```python
from build123d import *

# Parameters (mm, degrees)
F0_R     = 63.75
F1_DEPTH = 20
F2_R     = 55
F3_DEPTH = 25


with BuildPart() as f1:
    # F0 (on Top) → F1 (new body)
    with BuildSketch(Plane.XY):
        Circle(F0_R)
    extrude(amount=F1_DEPTH)


with BuildPart() as f3:
    # F2 (on Top) → F3 (new body)
    with BuildSketch(Plane.XY):
        with Locations((-173.995957, -105.135567)):
            Circle(F2_R)
    extrude(amount=F3_DEPTH)


with BuildPart() as f3_1:
    # F4: moved
    add(f3.part.moved(Location((173.8, 105.1, -2.2))))


with BuildPart() as f1_1:
    add(f1.part)

    # F5: cut F3
    add(f3_1.part, mode=Mode.SUBTRACT)


solid = f1_1.part
```
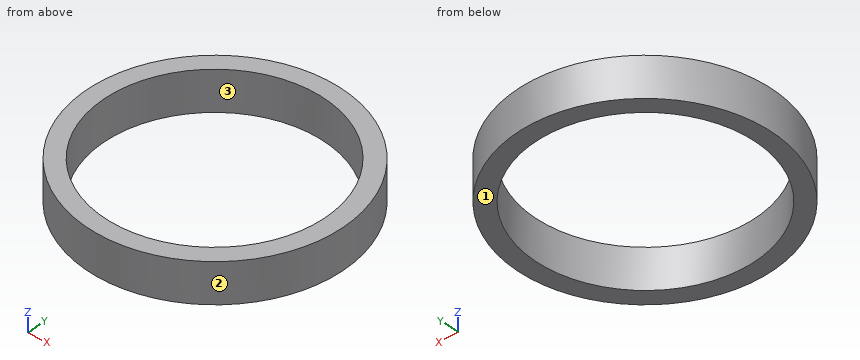
Check sheet for the modelled part. Datum: model origin and axes. Units: mm. Face numbers are marked on the shaded views. Coordinates: 2 decimals unless noted, no trailing zeros. Order: outer loops, then holes, each group sorted by start corner. A loop starts at its lowest first (then second) coordinate and runs counter-clockwise, first axis right, second up. Notation, with made-up numbers: (64.25, -5.5) -> (110.25, -5.5) arc R18 ccw to (110.25, 20.5) -> close; hole circle Ø9 at (34.25, 62.25). An arc over 180 degrees is marked (long way). Write item = value, one per line. Start each with the question number.
1) Cross-section at B-B (y = 29). Enter the section's corners in (x, z).
2) Go/stop test with flat-tipped pins: P1, Ø5, axis at y = -16.5, z = 17, coming from the +X side; P2, Ø2, axis at x = 43.5, z = 12, coming from the +Y side; P3, Ø5, axis at x = -13, z = 9.5, coming from the -Y side. Record where each tip stops, or that it passes through.
3) Cross-section at C-C (z = 9.25). Enter the section's corners in (x, y), then the cut area to 3 significant figures.
4) Mould release check, pull along Y, two halves, no side actions. Record for the marked faces 1, 2 and 3: +Y half, -Y half, draft (parallel to the pull), parting line (faces both ways), or undercut.
5) Cross-section at A-A (x = -26). Enter the section's corners in (y, z).
6) Material ranges on L1, parallel to Y at x = -1, z = 6.5; L2, parallel to X at y = 1.5, z = 2.25; L3, parallel to X at y = -43, z = 3.75, recorded low to high.
Ans:
q1.outline = (-56.77, 0) -> (-46.91, 0) -> (-46.91, 20) -> (-56.77, 20) -> close; (46.52, 0) -> (56.77, 0) -> (56.77, 20) -> (46.52, 20) -> close
q2.P1 = 62.19
q2.P2 = 47.52
q2.P3 = -62.88
q3.outline = circle Ø127.5 at (0, 0); hole circle Ø110 at (-0.2, -0.04)
q3.area = 3,260 mm²
q4.face_1 = draft
q4.face_2 = parting line
q4.face_3 = undercut
q5.outline = (-58.21, 0) -> (-48.61, 0) -> (-48.61, 20) -> (-58.21, 20) -> close; (48.54, 0) -> (58.21, 0) -> (58.21, 20) -> (48.54, 20) -> close
q6.L1 = -63.74 to -55.03, 54.96 to 63.74
q6.L2 = -63.73 to -55.17, 54.78 to 63.73
q6.L3 = -47.06 to -34.53, 34.14 to 47.06
